For this review, take the finished solid that the model builds, in its own axes (mm). Face numbers are marked on the shaded views. A direction names the side the tool comes from. Coordinates: 2 decimals unless noted, no trailing zeros. Loops run counter-clockwise (first coordinate to the right, second up) from the corner with the lowest first, then second, coordinate; pieces in that order, holes last. Notation, with made-up numbers: (88.25, -31.5) - (107.25, -31.5) arc R14 ccw to (107.25, -6.5) - close; hole circle Ø5 at (62.25, -10). An arc over 180 degrees is marked (long way). One line per item, written item: value. Start each with the question number.
1. Insertion check: pin 1 (2.5 mm diameter, centred on x = 15, z = 3, fed in from -Y); pin 2 (1.5 mm diameter, centred on x = 33.5, z = 3.5, fed in from +Y); pin 3 (13.5 mm diameter, centred on x = 25.5, y = 26, fed in from +Z). Each pin has a flat end and moves straight along its axis. Give the tip position at first contact, or say it passes through.
2. To check wall thickness, follow line 1 (X direction, y = -1.5, z = 1.25); line 2 (X direction, y = -5.5, z = 4.3); line 3 (X direction, y = 10, z = 2.55). State the ranges of each line that lie inside material, in increasing order. Write a range as from..to.
3. The part is to be moulded in two halves that separate along X. For the marked faces 4 and 5, say which applies: released by +X, released by -X, zero draft, split by the parting line, or undercut.
4. Take a section at A-A, the plane y = 0. State the section outline as (x, z) points.
5. Take a section at B-B, the plane x = 0. State the section outline as (y, z) points, and give its area (3 significant figures).
6. Take a section at C-C, the plane z = 3.95. State the section outline as (x, y) points, and give its area (3 significant figures).
7. For the marked faces 1, 2 and 3, list the 3-axis set-ups (+Z, -Z, +X, -X, +Y, -Y) from which the entire face can be reached by the end or side of a thin tool; tool diameter is ignored.
```python
from build123d import *

# Parameters (mm, degrees)
SKETCH_R        = 60
PAD_DEPTH       = 5
SKETCH001_W     = 12
SKETCH001_H     = 23
POCKET_DEPTH    = 4
FILLET_R        = 3
SKETCH002_W     = 24
SKETCH002_H     = 57
POCKET001_DEPTH = 3
SKETCH003_W     = 17
SKETCH003_H     = 25
SKETCH003_W_2   = 12
SKETCH003_H_2   = 20
POCKET002_DEPTH = 4.5
CHAMFER_SIZE    = 4


with BuildPart() as part:
    # Sketch → Pad (new body)
    with BuildSketch(Plane.XY):
        Circle(SKETCH_R)
    extrude(amount=PAD_DEPTH)

    # Sketch001 (on Face3 of Pad) → Pocket (cut)
    with BuildSketch(Plane.XY.offset(5)):
        with Locations((0, 5.9)):
            Rectangle(SKETCH001_W, SKETCH001_H)
    extrude(amount=-POCKET_DEPTH, mode=Mode.SUBTRACT)

    # Fillet
    fillet_edges = [part.edges().sort_by_distance(p)[0] for p in [
        (-60, 0, 5),
    ]]
    fillet(fillet_edges, radius=FILLET_R)

    # Sketch002 (on Face4 of Fillet) → Pocket001 (cut)
    with BuildSketch(Plane.XY.offset(5)):
        with Locations((25, -13.5)):
            Rectangle(SKETCH002_W, SKETCH002_H)
    extrude(amount=-POCKET001_DEPTH, mode=Mode.SUBTRACT)

    # Sketch003 (on Face4 of Pocket001) → Pocket002 (cut)
    with BuildSketch(Plane.XY.offset(5)):
        with Locations((25, 27.5)):
            Rectangle(SKETCH003_W, SKETCH003_H)
        with Locations((25, -52)):
            Rectangle(SKETCH003_W_2, SKETCH003_H_2)
    extrude(amount=-POCKET002_DEPTH, mode=Mode.SUBTRACT)

    # Chamfer
    chamfer_edges = [part.edges().sort_by_distance(p)[0] for p in [
        (25, 40, 5),
    ]]
    chamfer(chamfer_edges, length=CHAMFER_SIZE)


solid = part.part
```
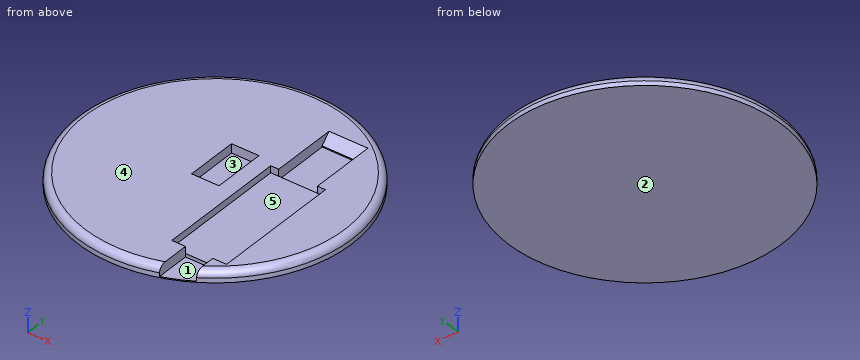
Solutions:
1. pin 1: y = -58.34
1. pin 2: y = 49.95
1. pin 3: z = 0.5
2. line 1: -59.98..-6, 6..59.98
2. line 2: -58.67..-6, 6..13, 37..58.67
2. line 3: -59.11..-6, 6..13, 37..59.11
3. face 4: zero draft
3. face 5: undercut
4. outline: (-60, 0) - (60, 0) - (60, 2) arc R3 ccw to (57, 5) - (37, 5) - (37, 2) - (13, 2) - (13, 5) - (6, 5) - (6, 1) - (-6, 1) - (-6, 5) - (-57, 5) arc R3 ccw to (-60, 2) - close
5. outline: (-60, 0) - (60, 0) - (60, 2) arc R3 ccw to (57, 5) - (17.4, 5) - (17.4, 1) - (-5.6, 1) - (-5.6, 5) - (-57, 5) arc R3 ccw to (-60, 2) - close
5. area: 504 mm2
6. outline: (13, -42) - (13, 15) - (16.5, 15) - (16.5, 42.95) - (33.5, 42.95) - (33.5, 15) - (37, 15) - (37, -42) - (31, -42) - (31, -50.53) arc R59.28 ccw (long way) to (19, -56.15) - (19, -42) - close; hole (-6, -5.6) - (6, -5.6) - (6, 17.4) - (-6, 17.4) - close
6. area: 8,780 mm2
7. face 1: +Z, -Y
7. face 2: -Z, +X, -X, +Y, -Y
7. face 3: +Z
